Autodesk Inventor part; units mm, degrees
ref_plane "Work Plane1" through (0, 100, 0) normal (0, 1, 0) x (-1, 0, 0)
ref_plane "YZ Plane" through (0, 0, 0) normal (1, 0, 0) x (0, 1, 0)
ref_plane "XY Plane" through (0, 0, 0) normal (0, 0, 1) x (1, 0, 0)
sketch "Sketch1" plane through (0, 0, 0) normal (0, 0, 1) x (1, 0, 0)
  line L0 (0, 0) -> (0, 275)
  line L1 (25, 300) -> (255, 300)
  line L2 (280, 275) -> (280, 180)
  line L3 (280, 180) -> (435, 180)
  line L4 (460, 155) -> (460, 0)
  arc A0 (25, 300) -> (0, 275) centre (25, 275) ccw
  arc A1 (280, 275) -> (255, 300) centre (255, 275) ccw
  arc A2 (460, 155) -> (435, 180) centre (435, 155) ccw
  line L5 (280, 180) -> (280, 93.2639)
  point P0 (0, 300)
  point P1 (280, 300)
  point P2 (460, 180)
  dimension "d0" = 300
  dimension "d1" = 280
  dimension "d2" = 120
  dimension "d3" = 180
  dimension "d4" = 25
  dimension "d5" = 25
  dimension "d6" = 25
  dimension "d7" = 86.7361
sketch "Sketch2" plane through (0, 0, 0) normal (0, 1, 0) x (-1, 0, 0)
  circle A0 centre (0, 0) radius 11.25
  dimension "d8" = 22.5
sweep "Sweep1" add profiles "Sketch2" path "Sketch1" path curves L0 A0 L1 A1 L2 L3 A2 L4
sketch "Sketch3" plane through (0, 0, 0) normal (0, 1, 0) x (-1, 0, 0)
  point P0 (0, 0)
sketch "Sketch4" plane through (0, 0, 0) normal (0, 0, 1) x (1, 0, 0)
  line L0 (280, 180) -> (280, 180)
  line L1 (280, 180) -> (280, 100)
  point P0 (0, 0)
  dimension "d11" = 80
ref_plane "Work Plane1" through (0, 100, 0) normal (0, 1, 0) x (-1, 0, 0)
sketch "Sketch5" plane through (0, 100, 0) normal (0, 1, 0) x (-1, 0, 0)
  circle A0 centre (-280, 0) radius 11.25
  circle A1 centre (-280, 0) radius 11.25
  point P0 (0, 0)
  dimension "d13" = 22.5
sweep "Sweep2" add profiles "Sketch5" path "Sketch4" path curves L1
sketch "Sketch6" plane through (0, 0, 0) normal (0, 0, 1) x (1, 0, 0)
  line L0 (0, 101.8033) -> (281.8033, 101.8033)
  line L1 (281.8033, 101.8033) -> (281.8033, 221.8033)
  line L2 (281.8033, 221.8033) -> (0, 221.8033)
  line L3 (0, 221.8033) -> (0, 101.8033)
  point P0 (0, 0)
  dimension "d16" = 120
extrude "Extrusion1" add sketch "Sketch6" along normal blind 2.5
properties part number "frame of armrest"
Verification items for the finished model (mm, model axes). A direction names the side the tool comes from. Coordinates: 2 decimals unless noted, no trailing zeros. Loops run counter-clockwise (first coordinate to the right, second up) from the corner with the lowest first, then second, coordinate; pieces in that order, holes last. Notation, with made-up numbers: (-33.75, 48.5) - (-18.75, 48.5) arc R20 cw to (-18.75, 69.5) - close; hole circle Ø9 at (9, 56.25). An arc over 180 degrees is marked (long way). Put each result on its own line as item: value.
Item 1: Set-up check for faces 3 (the face through (270.649, 186.275, 6.255)), 4 (the face through (448.76, 76.41, 0.49)), 5 (the face through (138, 163, 2.5)): record each of +Z, -Z, +X, -X, +Y, -Y from which the full face is reachable in a straight line by a thin tool's end or side.
Conclusion:
face 3: none
face 4: -Y
face 5: +Z, -Y
Item 2: Draft check along X on faces 1 (the face through (280, 100, 0)), 2 (the face through (0, 0, 0)). Enter one of: pulls with the +X half, pulls with the -X half, needs draft (parallel to the pull), parting line crosses it, or undercut.
Conclusion:
face 1: undercut
face 2: needs draft
Item 3: Section check D-D (y = 201.5). Enter the section's corners in (x, z), then the cut area to 3 significant figures.
Conclusion:
outline: (10.97, 2.5) arc R11.25 ccw (long way) to (11.25, 0) - (268.75, 0) arc R11.25 ccw (long way) to (269.03, 2.5) - close
area: 1,440 mm2
Item 4: Gauge pin test, flat ends, axial feed: pin 1 Ø3 at (x, z) = (166.5, 2) entering from -Y; pin 2 Ø4 at (y, z) = (274, -3) entering from +X; pin 3 Ø6 at (x, z) = (320, -0.5) entering from -Y; pin 4 Ø2 at (x, z) = (176.5, 1) entering from +Y. Record the tip position at first contact, or that the pin passes through.
Conclusion:
pin 1: stops at y = 101.8
pin 2: stops at x = 291.21
pin 3: stops at y = 168.75
pin 4: stops at y = 311.25
Item 5: Section check A-A (y = 250). Enter the section's corners in (x, z), then the cut area to 3 significant figures.
Conclusion:
outline: circle Ø22.5 at (0, 0); circle Ø22.5 at (280, 0)
area: 795 mm2
Item 6: Section check B-B (x = 101). Enter the section's corners in (y, z), then the cut area to 3 significant figures.
Conclusion:
outline: (101.8, 0) - (221.8, 0) - (221.8, 2.5) - (101.8, 2.5) - close; circle Ø22.5 at (300, 0)
area: 698 mm2
Item 7: Scan lines: line 1 along X through (y, z) = (147, -3.75); line 2 along X through (y, z) = (147, -4.5); line 3 along X through (y, z) = (77.5, -1.25). Record each from-to range of solid material in increasing order.
Conclusion:
line 1: x = -10.61 to 10.61, 269.39 to 290.61, 449.39 to 470.61
line 2: x = -10.31 to 10.31, 269.69 to 290.31, 449.69 to 470.31
line 3: x = -11.18 to 11.18, 448.82 to 471.18
Item 8: Section check C-C (z = 7). Enter the section's corners in (x, y).
Conclusion:
outline: (-8.81, 0) - (8.81, 0) - (8.81, 275) arc R16.19 cw to (25, 291.19) - (255, 291.19) arc R16.19 cw to (271.19, 275) - (271.19, 100) - (288.81, 100) - (288.81, 171.19) - (435, 171.19) arc R16.19 cw to (451.19, 155) - (451.19, 0) - (468.81, 0) - (468.81, 155) arc R33.81 ccw to (435, 188.81) - (288.81, 188.81) - (288.81, 275) arc R33.81 ccw to (255, 308.81) - (25, 308.81) arc R33.81 ccw to (-8.81, 275) - close
